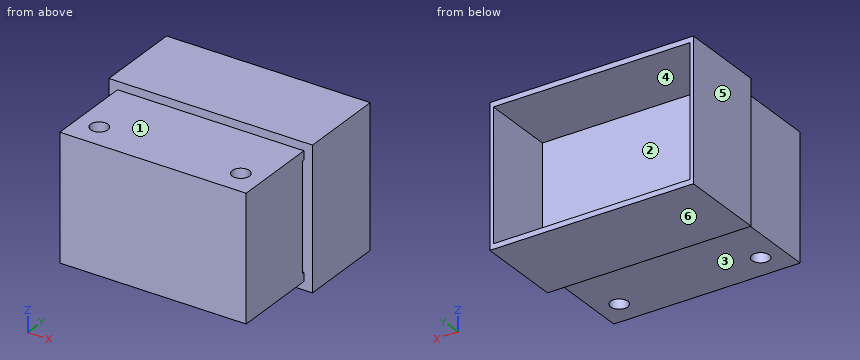
Autodesk Inventor part; units mm, degrees
ref_plane "YZ Plane" through (0, 0, 0) normal (1, 0, 0) x (0, 1, 0)
ref_plane "XZ Plane" through (0, 0, 0) normal (0, 1, 0) x (-1, 0, 0)
ref_plane "XY Plane" through (0, 0, 0) normal (0, 0, 1) x (1, 0, 0)
sketch "Sketch1" plane through (0, 0, 0) normal (0, 1, 0) x (-1, 0, 0)
  point P0 (0, 0)
sketch "Sketch2" plane through (0, 0, 0) normal (0, 1, 0) x (-1, 0, 0)
  line L0 (-10.7689, -7.215) -> (10.7689, -7.215)
  line L1 (10.7689, -7.215) -> (10.7689, 7.215)
  line L2 (10.7689, 7.215) -> (-10.7689, 7.215)
  line L3 (-10.7689, 7.215) -> (-10.7689, -7.215)
  line L4 (-10.7689, -7.215) -> (10.7689, 7.215) construction
  line L5 (10.7689, -7.215) -> (-10.7689, 7.215) construction
  line L6 (9.5058, 5.9518) -> (9.5058, -5.9518)
  line L7 (9.5058, -5.9518) -> (-9.5058, -5.9518)
  line L8 (-9.5058, -5.9518) -> (-9.5058, 5.9518)
  line L9 (-9.5058, 5.9518) -> (9.5058, 5.9518)
  point P0 (0, 0)
extrude "Extrusion1" add sketch "Sketch2" along normal blind 10
sketch "Sketch3" plane through (-10.7689, 0, 7.215) normal (0, 0, 1) x (1, 0, 0)
  circle A0 centre (2.5905, 2.9643) radius 1
  line L0 (20.2747, 10) -> (1.2632, 10)
  line L1 (10.7689, 10) -> (10.7689, 0)
  circle A1 centre (18.9473, 2.9643) radius 1
  dimension "d2" = 2
extrude "Extrusion2" cut sketch "Sketch3" against normal through all
extrude "Extrusion3" add sketch "Sketch2" along normal blind 1 contours L6 L7 L8 L9
sketch "Sketch4" plane through (10.7689, 0, 7.215) normal (1, 0, 0) x (0, 0, -1)
  line L0 (0, 0) -> (14.4299, 0)
  line L1 (14.4299, 0) -> (14.4299, 10)
  line L2 (0, 10) -> (14.4299, 10)
  line L3 (0, 0) -> (0, 10)
  point P0 (7.215, 0)
sketch "Sketch5" plane through (0, 10, 0) normal (0, 1, 0) x (1, 0, 0)
  line L0 (-9.5058, -5.9518) -> (-9.5058, 5.9518)
  line L1 (-9.5058, 5.9518) -> (9.5058, 5.9518)
  line L2 (9.5058, 5.9518) -> (9.5058, -5.9518)
  line L3 (9.5058, -5.9518) -> (-9.5058, -5.9518)
  line L4 (-9.7558, 6.2018) -> (-9.7558, -6.2018)
  line L5 (-9.7558, -6.2018) -> (9.7558, -6.2018)
  line L6 (9.7558, -6.2018) -> (9.7558, 6.2018)
  line L7 (9.7558, 6.2018) -> (-9.7558, 6.2018)
  point P0 (0, 0)
  dimension "d8" = 0.25
extrude "Extrusion4" cut sketch "Sketch5" against normal blind 0.25
sketch "Sketch6" plane through (9.7558, 10, -6.2018) normal (-1, 0, 0) x (0, 0, 1)
  line L0 (0, 0) -> (12.4036, 0)
  line L1 (0, 0) -> (0, -0.25)
  line L2 (0, -0.25) -> (12.4036, -0.25)
  line L3 (12.4036, 0) -> (12.4036, -0.25)
  point P0 (6.2018, -10)
sketch "Sketch7" plane through (10.7689, 0, 7.215) normal (1, 0, 0) x (0, 0, -1)
  line L0 (0, 10) -> (14.4299, 10)
  line L1 (1.0132, 10) -> (1.0132, 9.75)
  line L2 (13.4167, 10) -> (1.0132, 10)
  line L3 (1.0132, 10) -> (13.4167, 10)
  line L4 (1.0132, 10) -> (13.4167, 10)
  line L5 (1.0132, 10) -> (1.0132, 9.75)
  line L6 (1.0132, 9.75) -> (13.4167, 9.75)
  line L7 (13.4167, 9.75) -> (13.4167, 10)
  line L8 (13.4167, 10) -> (1.0132, 10)
  line L9 (1.0132, 10) -> (13.4167, 10)
  line L10 (13.4167, 10) -> (13.4167, 9.75)
  line L11 (13.4167, 9.75) -> (1.0132, 9.75)
  line L12 (1.0132, 9.75) -> (1.0132, 10)
  point P0 (7.215, 0)
  dimension "d11" = 0.25
extrude "Extrusion5" cut sketch "Sketch7" against normal up to surface (1.0132 mm away)
sketch "Sketch8" plane through (0, 10, 0) normal (0, 1, 0) x (1, 0, 0)
  line L0 (11.7647, -8.1506) -> (-11.7647, -8.1506)
  line L1 (-11.7647, -8.1506) -> (-11.7647, 8.1506)
  line L2 (-11.7647, 8.1506) -> (11.7647, 8.1506)
  line L3 (11.7647, 8.1506) -> (11.7647, -8.1506)
  line L4 (11.7647, -8.1506) -> (-11.7647, 8.1506) construction
  line L5 (-11.7647, -8.1506) -> (11.7647, 8.1506) construction
  line L6 (11.3506, -7.5482) -> (-11.3506, -7.5482)
  line L7 (-11.3506, -7.5482) -> (-11.3506, 7.5482)
  line L8 (-11.3506, 7.5482) -> (11.3506, 7.5482)
  line L9 (11.3506, 7.5482) -> (11.3506, -7.5482)
  line L10 (11.3506, -7.5482) -> (-11.3506, 7.5482) construction
  line L11 (-11.3506, -7.5482) -> (11.3506, 7.5482) construction
  point P0 (0, 0)
extrude "Extrusion6" add sketch "Sketch8" along normal blind 10
sketch "Sketch9" plane through (0, 10, 0) normal (0, 1, 0) x (1, 0, 0)
  line L0 (-9.7558, 6.2018) -> (10.7689, 6.2018)
  line L1 (10.7689, 6.2018) -> (10.7689, 7.215)
  line L2 (10.7689, 7.215) -> (-10.7689, 7.215)
  line L3 (-10.7689, 7.215) -> (-10.7689, -7.215)
  line L4 (-10.7689, -7.215) -> (10.7689, -7.215)
  line L5 (10.7689, -7.215) -> (10.7689, -6.2018)
  line L6 (10.7689, -6.2018) -> (-9.7558, -6.2018)
  line L7 (-9.7558, -6.2018) -> (-9.7558, 6.2018)
  line L8 (10.7689, -7.215) -> (-10.7689, -7.215)
  line L9 (-10.7689, -7.215) -> (-10.7689, 7.215)
  line L10 (-10.7689, 7.215) -> (10.7689, 7.215)
  line L11 (10.7689, 7.215) -> (10.7689, -7.215)
  line L12 (10.7689, -7.215) -> (-10.7689, 7.215) construction
  line L13 (-10.7689, -7.215) -> (10.7689, 7.215) construction
  point P0 (0, 0)
extrude "Extrusion7" add sketch "Sketch8" along normal blind 1.5 contours L6 L7 L8 L9
properties part number "base_box"
Geometry: final body of the model. Coordinates: model frame, mm. Face numbers are marked on the shaded views. A direction names the side the tool comes from. Round coordinates to 2 decimals unless told otherwise and drop trailing zeros. Order: outer loops, then holes, each group sorted by start corner. A loop starts at its lowest first (then second) coordinate and runs counter-clockwise, first axis right, second up.
Q1. Section A-A, the plane x = 1.5. Output: boundary loops of the cut face in (y, z) (3 decimals), and give its area (3 significant figures).
Result sheet:
outline: (0, -7.215) - (10, -7.215) - (10, -8.151) - (20, -8.151) - (20, -7.548) - (11.5, -7.548) - (11.5, 7.548) - (20, 7.548) - (20, 8.151) - (10, 8.151) - (10, 7.215) - (0, 7.215) - close; hole (1, -5.952) - (9.75, -5.952) - (9.75, -6.202) - (10, -6.202) - (10, 6.202) - (9.75, 6.202) - (9.75, 5.952) - (1, 5.952) - close
area: 71.7 mm2
Q2. Access query for the marked faces 1, 2 and 3. Directions: +Z, -Z, +X, -X, +Y, -Y. A direction counts if a zero-diameter tool reaches every point of the face in a straight line with its end or side. Return the directions, or none.
Result sheet:
face 1: +Z, +X, -X, -Y
face 2: +Y
face 3: -Z, +X, -X, -Y
Q3. Mould query, pull axis X, two halves, no side actions, for the marked faces 4, 5 and 6. Classes: released by +X, released by -X, zero draft, split by the parting line, or undercut.
Result sheet:
face 4: undercut
face 5: released by -X
face 6: zero draft
Q4. Section C-C, the plane z = -0.5. Output: boundary loops of the cut face in (x, y), and give its area (3 significant figures).
Result sheet:
outline: (-11.76, 10) - (-10.77, 10) - (-10.77, 0) - (10.77, 0) - (10.77, 9.75) - (9.51, 9.75) - (9.51, 1) - (-9.51, 1) - (-9.51, 9.75) - (-9.76, 9.75) - (-9.76, 10) - (11.76, 10) - (11.76, 20) - (11.35, 20) - (11.35, 11.5) - (-11.35, 11.5) - (-11.35, 20) - (-11.76, 20) - close
area: 86.2 mm2
Q5. Material intervals for probe 1 along X at (y, z) = (15.25, 3.25); probe 2 along Z at (x, y) = (-3.75, 16); probe 3 along Y at (x, z) = (-7.75, 1.5), sorted ascending.
Result sheet:
probe 1: x = -11.76 to -11.35, 11.35 to 11.76
probe 2: z = -8.15 to -7.55, 7.55 to 8.15
probe 3: y = 0 to 1, 10 to 11.5
Q6. Pin query (flat end, axial travel): pin 1 (1.8 mm diameter, centred on x = 8.18, y = 2.96, fed in from +Z); pin 2 (2.5 mm diameter, centred on y = 4, z = 1.5, fed in from +X); pin 3 (3 mm diameter, centred on y = 3, z = 2, fed in from -X); pin 4 (5 mm diameter, centred on x = 0, y = 4, fed in from +Z) (3 decimals). Return the tip coordinate at first contact, or that it passes through.
Result sheet:
pin 1: passes through
pin 2: stops at x = 10.77
pin 3: stops at x = -10.77
pin 4: stops at z = 7.215
Q7. Section D-D, the plane y = 8. Output: boundary loops of the cut face in (x, z) (3 decimals), and give its area (3 significant figures).
Result sheet:
outline: (-10.769, -7.215) - (10.769, -7.215) - (10.769, 7.215) - (-10.769, 7.215) - close; hole (-9.506, -5.952) - (9.506, -5.952) - (9.506, 5.952) - (-9.506, 5.952) - close
area: 84.5 mm2
Q8. Section B-B, the plane y = 17.5. Output: boundary loops of the cut face in (x, z).
Result sheet:
outline: (-11.76, -8.15) - (11.76, -8.15) - (11.76, 8.15) - (-11.76, 8.15) - close; hole (-11.35, -7.55) - (11.35, -7.55) - (11.35, 7.55) - (-11.35, 7.55) - close
